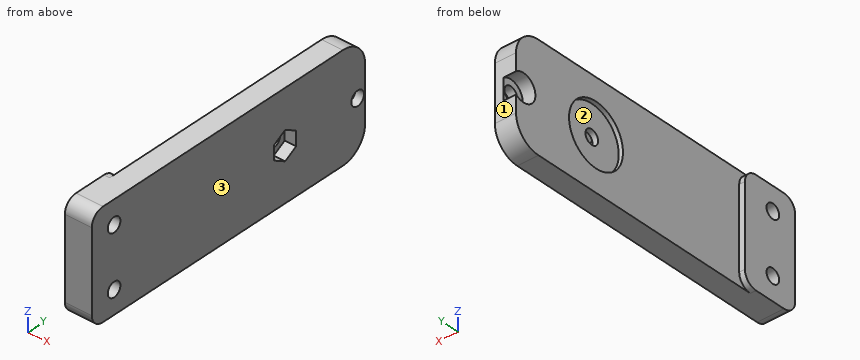
from build123d import *

# Parameters (mm, degrees)
COVER_START       = -26.9
COVER_PLATE_DEPTH = 5
TAIL_START        = -28.25
TAIL_PAD_DEPTH    = 1.55
PIN_START         = -27.1
SKETCH3_R         = 7.25
PIN_SEAT_DEPTH    = 1.2
BOLT_START        = -28.55
SKETCH4_R         = 1.7
BOLT_HOLES_DEPTH  = 6.85
PIN_START_2       = -24.6
PIN_NUT_DEPTH     = 2.9
COUNTERBORE_START = -27.1
SKETCH6_R         = 3.2
COUNTERBORE_DEPTH = 3.2


with BuildPart() as part:
    # Sketch1 → Cover plate (new body)
    with BuildSketch(Plane(origin=(0, 0, 0), x_dir=(0, 0, -1), z_dir=(1, 0, 0)).offset(COVER_START)):
        with BuildLine():
            Line((-1.5, 271.5), (-1.5, 336))
            ThreePointArc((-1.5, 336), (-3.257359313, 340.242640687), (-7.5, 342))
            Line((-7.5, 342), (-20.5, 342))
            ThreePointArc((-20.5, 342), (-24.742640687, 340.242640687), (-26.5, 336))
            Line((-26.5, 336), (-26.5, 271.5))
            ThreePointArc((-26.5, 271.5), (-25.621320344, 269.378679656), (-23.5, 268.5))
            Line((-23.5, 268.5), (-4.5, 268.5))
            ThreePointArc((-4.5, 268.5), (-2.378679656, 269.378679656), (-1.5, 271.5))
        make_face()
    extrude(amount=COVER_PLATE_DEPTH)

    # Sketch2 → Tail pad (add)
    with BuildSketch(Plane(origin=(0, 0, 0), x_dir=(0, 0, -1), z_dir=(1, 0, 0)).offset(TAIL_START)):
        with BuildLine():
            Line((-1.5, 271.5), (-1.5, 279))
            ThreePointArc((-1.5, 279), (-2.378679656, 281.121320344), (-4.5, 282))
            Line((-4.5, 282), (-23.5, 282))
            ThreePointArc((-23.5, 282), (-25.621320344, 281.121320344), (-26.5, 279))
            Line((-26.5, 279), (-26.5, 271.5))
            ThreePointArc((-26.5, 271.5), (-25.621320344, 269.378679656), (-23.5, 268.5))
            Line((-23.5, 268.5), (-4.5, 268.5))
            ThreePointArc((-4.5, 268.5), (-2.378679656, 269.378679656), (-1.5, 271.5))
        make_face()
    extrude(amount=TAIL_PAD_DEPTH)

    # Sketch3 → Pin seat (cut)
    with BuildSketch(Plane(origin=(0, 0, 0), x_dir=(0, 0, -1), z_dir=(1, 0, 0)).offset(PIN_START)):
        with Locations((-14, 320.5)):
            Circle(SKETCH3_R)
    extrude(amount=PIN_SEAT_DEPTH, mode=Mode.SUBTRACT)

    # Sketch4 → Bolt holes (cut)
    with BuildSketch(Plane(origin=(0, 0, 0), x_dir=(0, 0, -1), z_dir=(1, 0, 0)).offset(BOLT_START)):
        with Locations((-14, 320.5)):
            Circle(SKETCH4_R)
        with Locations((-7, 274.5)):
            Circle(SKETCH4_R)
        with Locations((-21, 274.5)):
            Circle(SKETCH4_R)
        with Locations((-14, 340)):
            Circle(SKETCH4_R)
    extrude(amount=BOLT_HOLES_DEPTH, mode=Mode.SUBTRACT)

    # Sketch5 → Pin nut (cut)
    with BuildSketch(Plane(origin=(0, 0, 0), x_dir=(0, 0, -1), z_dir=(1, 0, 0)).offset(PIN_START_2)):
        Polygon((-15.703183294, 323.45), (-17.406366588, 320.5), (-15.703183294, 317.55), (-12.296816706, 317.55), (-10.593633412, 320.5), (-12.296816706, 323.45), align=None)
    extrude(amount=PIN_NUT_DEPTH, mode=Mode.SUBTRACT)

    # Sketch6 → Counterbore (cut)
    with BuildSketch(Plane(origin=(0, 0, 0), x_dir=(0, 0, -1), z_dir=(1, 0, 0)).offset(COUNTERBORE_START)):
        with Locations((-14, 340)):
            Circle(SKETCH6_R)
    extrude(amount=COUNTERBORE_DEPTH, mode=Mode.SUBTRACT)


solid = part.part
For this review, take the finished solid that the model builds, in its own axes (mm). Face numbers are marked on the shaded views. Round coordinates to 2 decimals unless told otherwise and drop trailing zeros. Order: outer loops, then holes, each group sorted by start corner. A loop starts at its lowest first (then second) coordinate and runs counter-clockwise, first axis right, second up. Notation, with made-up numbers: M -29,-33 L 29,-33 A21 cw 29,-18 Z; hole C 60.5,-6 d5. An arc over 180 degrees is marked long. Use a Markdown table: item, result. Add a question column.
Item 1: Add section B-B, the plane x = -22.75. Give the boundary of the cut face in (y, z), then the cut area to 3 significant figures.
Item 2: Add section D-D, the plane y = 340. Give the boundary of the cut face in (x, z), then the cut area to 3 significant figures.
Item 3: Add section A-A, the plane z = 14. Give the boundary of the cut face in (x, y).
Item 4: Insertion check: pin 1 (5.5 mm diameter, centred on y = 320.5, z = 14, fed in from +X); pin 2 (4 mm diameter, centred on y = 340, z = 14, fed in from -X); pin 3 (5.5 mm diameter, centred on y = 339.5, z = 13.5, fed in from -X); pin 4 (2 mm diameter, centred on y = 274.5, z = 7, fed in from -X). Each pin has a flat end and moves straight along its axis. Give the tip position at first contact, or say it passes through.
Item 5: Add section C-C, the plane y = 274.5. Give the boundary of the cut face in (x, z).
Item 6: Mouldability with a two-part tool opening along Y and no side actions: class the marked faces 1, 2 and 3 as released by +Y, released by -Y, zero draft, split by the parting line, or undercut.
Item 7: To check wall thickness, follow line 1 along Y through (x, z) = (-23.4, 14); line 2 along Z through (x, y) = (-25.25, 274.5); line 3 along Y through (x, z) = (-27.5, 23.5). State the ranges of each line that lie inside material, in increasing order.
Geometry results:
| question | item | result |
|---|---|---|
| 1 | outline | M 268.5,4.5 A3 ccw 271.5,1.5 L 336,1.5 A6 ccw 342,7.5 L 342,20.5 A6 ccw 336,26.5 L 271.5,26.5 A3 ccw 268.5,23.5 Z; hole C 274.5,7 d3.4; hole C 274.5,21 d3.4; hole M 317.55,12.3 L 320.5,10.59 L 323.45,12.3 L 323.45,15.7 L 320.5,17.41 L 317.55,15.7 Z; hole C 340,14 d3.4 |
| 1 | area | 1,760 mm² |
| 2 | outline | M -26.9,3.03 L -21.9,3.03 L -21.9,12.3 L -23.9,12.3 L -23.9,10.8 L -26.9,10.8 Z; M -26.9,17.2 L -23.9,17.2 L -23.9,15.7 L -21.9,15.7 L -21.9,24.97 L -26.9,24.97 Z |
| 2 | area | 83.7 mm² |
| 3 | outline | M -28.25,268.5 L -21.9,268.5 L -21.9,317.55 L -24.6,317.55 L -24.6,318.8 L -25.9,318.8 L -25.9,313.25 L -26.9,313.25 L -26.9,282 L -28.25,282 Z; M -26.9,327.75 L -25.9,327.75 L -25.9,322.2 L -24.6,322.2 L -24.6,323.45 L -21.9,323.45 L -21.9,338.3 L -23.9,338.3 L -23.9,336.8 L -26.9,336.8 Z; M -23.9,341.7 L -21.9,341.7 L -21.9,342 L -23.9,342 Z |
| 4 | pin 1 | stops at x = -24.6 |
| 4 | pin 2 | stops at x = -23.9 |
| 4 | pin 3 | stops at x = -26.9 |
| 4 | pin 4 | passes through |
| 5 | outline | M -28.25,1.5 L -21.9,1.5 L -21.9,5.3 L -28.25,5.3 Z; M -28.25,8.7 L -21.9,8.7 L -21.9,19.3 L -28.25,19.3 Z; M -28.25,22.7 L -21.9,22.7 L -21.9,26.5 L -28.25,26.5 Z |
| 6 | face 1 | released by +Y |
| 6 | face 2 | undercut |
| 6 | face 3 | zero draft |
| 7 | line 1 | y = 268.5 to 317.55, 323.45 to 338.3, 341.7 to 342 |
| 7 | line 2 | z = 1.5 to 5.3, 8.7 to 19.3, 22.7 to 26.5 |
| 7 | line 3 | y = 268.5 to 282 |
